from build123d import *

# Parameters (mm, degrees)
SKETCH2_OUTSIDE_W  = 35.136
SKETCH2_OUTSIDE_H  = 35.136
SKETCH2_OUTSIDE_R  = 2.1082
CUT_EXTRUDE1_DEPTH = 22.020706078


with BuildPart() as part:
    # Sketch1 → Revolve1 (revolve)
    with BuildSketch(Plane(origin=(0, 0, 0), x_dir=(0, 0, -1), z_dir=(1, 0, 0)), mode=Mode.PRIVATE) as revolve1_sk:
        Polygon((-0.254, 5.5626), (10.922, 5.5626), (10.922, 4.24942), (9.906, 4.24942), (9.724157759, 4.56438), (-3.429, 4.56438), (-3.429, 12.7), (-0.254, 12.7), align=None)
    revolve(revolve1_sk.sketch.rotate(Axis((0, 0, -8.471806123), (0, 0, -1)), 90), axis=Axis((0, 0, -8.471806123), (0, 0, -1)))

    # Sketch2 outside → Cut-Extrude1 (cut, through all)
    # profile 1 of 3: a face of its own
    with BuildSketch(Plane.XY):
        Rectangle(SKETCH2_OUTSIDE_W, SKETCH2_OUTSIDE_H)
        with BuildLine():
            Line((6.607062287, 2.733250436), (3.520637098, 10.194038953))
            ThreePointArc((3.520637098, 10.194038953), (0, 12.5476), (-3.520637098, 10.194038953))
            Line((-3.520637098, 10.194038953), (-6.607062287, 2.733250436))
            ThreePointArc((-6.607062287, 2.733250436), (-7.1501, 0), (-6.607062287, -2.733250436))
            Line((-6.607062287, -2.733250436), (-3.520637098, -10.194038953))
            ThreePointArc((-3.520637098, -10.194038953), (0, -12.5476), (3.520637098, -10.194038953))
            Line((3.520637098, -10.194038953), (6.607062287, -2.733250436))
            ThreePointArc((6.607062287, -2.733250436), (7.1501, 0), (6.607062287, 2.733250436))
        make_face(mode=Mode.SUBTRACT)
    # profile 2 of 3: a face of its own
    with BuildSketch(Plane.XY):
        with Locations((0, 8.7376)):
            Circle(SKETCH2_OUTSIDE_R)
    # profile 3 of 3: a face of its own
    with BuildSketch(Plane.XY):
        with Locations((0, -8.7376)):
            Circle(SKETCH2_OUTSIDE_R)
    extrude(amount=CUT_EXTRUDE1_DEPTH, mode=Mode.SUBTRACT)


solid = part.part
Could you check a few things on this model? Use its own coordinates, in mm. A direction names the side the tool comes from. Give positions to 0.01 mm unless a question says otherwise; leave off trailing zeros. Order: outer loops, then holes, each group sorted by start corner. A loop starts at its lowest first (then second) coordinate and runs counter-clockwise, first axis right, second up.
Item 1: I'm going to push flat-ended pins straight in: pin 1 (4 mm diameter, centred on y = -6, z = -4, fed in from +X); pin 2 (5 mm diameter, centred on x = -0.5, z = -5, fed in from +Y); pin 3 (5 mm diameter, centred on y = 2.5, z = -5.5, fed in from -X). Where does each tip first touch, or does it pass through?
Item 2: If we section it at D-D, the plane z = -0.75: Write out the boundary of the cut face in (x, y), plus the area to 3 significant figures.
Item 3: If we mould it in two halves opening along Y, with no side actions, what happens to faces 1 (the face through (-0.274, -6.647, 1.819)), 2 (the face through (5.306, -1.671, -5.412)), 3 (the face through (-5, -3, 0.254)), 4 (the face through (4.05, -1.28, -10.41))? For each: pulls with the +Y half, pulls with the -Y half, needs draft (parallel to the pull), parting line crosses it, or undercut.
Item 4: I need wall thicknesses on line 1 (Y direction, x = 0, z = 2.5); line 2 (Y direction, x = 0, z = -6.5); line 3 (Z direction, x = 2, y = -9.5). Which ranges of each line are inside material? Lowest first, please.
Item 5: If we section it at A-A, the plane y = 0: Write out the boundary of the cut face in (x, z), plus the area to 3 significant figures.
Item 6: If we section it at B-B, the plane x = 0: Write out the boundary of the cut face in (y, z), plus the area to 3 significant figures.
Item 7: For faces 5 (the face through (-7.15, 0.04, 1.82)), 6 (the face through (-4.56, -0.2, -3.06)), which set-ups out of +Z, -Z, +X, -X, +Y, -Y let a thin tool reach every point of the face, with its end or its side?
Item 8: If we section it at C-C, the plane z = 1.5: Write out the boundary of the cut face in (x, y), plus the area to 3 significant figures.
Values:
1. pin 1: stops at x = 3.87
1. pin 2: stops at y = 5.56
1. pin 3: stops at x = -5.56
2. outline: circle Ø11.13 at (0, 0); hole circle Ø9.13 at (0, 0)
2. area: 31.8 mm2
3. face 1: undercut
3. face 2: parting line crosses it
3. face 3: needs draft
3. face 4: undercut
4. line 1: y = -12.55 to -10.85, -6.63 to -4.56, 4.56 to 6.63, 10.85 to 12.55
4. line 2: y = -5.56 to -4.56, 4.56 to 5.56
4. line 3: z = 0.25 to 3.43
5. outline: (-7.15, 0.25) - (-5.56, 0.25) - (-5.56, -10.92) - (-4.25, -10.92) - (-4.25, -9.91) - (-4.56, -9.72) - (-4.56, 3.43) - (-7.15, 3.43) - close; (4.25, -10.92) - (5.56, -10.92) - (5.56, 0.25) - (7.15, 0.25) - (7.15, 3.43) - (4.56, 3.43) - (4.56, -9.72) - (4.25, -9.91) - close
5. area: 39.4 mm2
6. outline: (-12.55, 0.25) - (-10.85, 0.25) - (-10.85, 3.43) - (-12.55, 3.43) - close; (-6.63, 0.25) - (-5.56, 0.25) - (-5.56, -10.92) - (-4.25, -10.92) - (-4.25, -9.91) - (-4.56, -9.72) - (-4.56, 3.43) - (-6.63, 3.43) - close; (4.25, -10.92) - (5.56, -10.92) - (5.56, 0.25) - (6.63, 0.25) - (6.63, 3.43) - (4.56, 3.43) - (4.56, -9.72) - (4.25, -9.91) - close; (10.85, 0.25) - (12.55, 0.25) - (12.55, 3.43) - (10.85, 3.43) - close
6. area: 46.9 mm2
7. face 5: +Z, -Z, -X
7. face 6: +Z
8. outline: (-6.61, -2.73) - (-3.52, -10.19) arc R3.81 ccw to (3.52, -10.19) - (6.61, -2.73) arc R7.15 ccw to (6.61, 2.73) - (3.52, 10.19) arc R3.81 ccw to (-3.52, 10.19) - (-6.61, 2.73) arc R7.15 ccw to start; hole circle Ø9.13 at (0, 0); hole circle Ø4.22 at (0, -8.74); hole circle Ø4.22 at (0, 8.74)
8. area: 158 mm2
